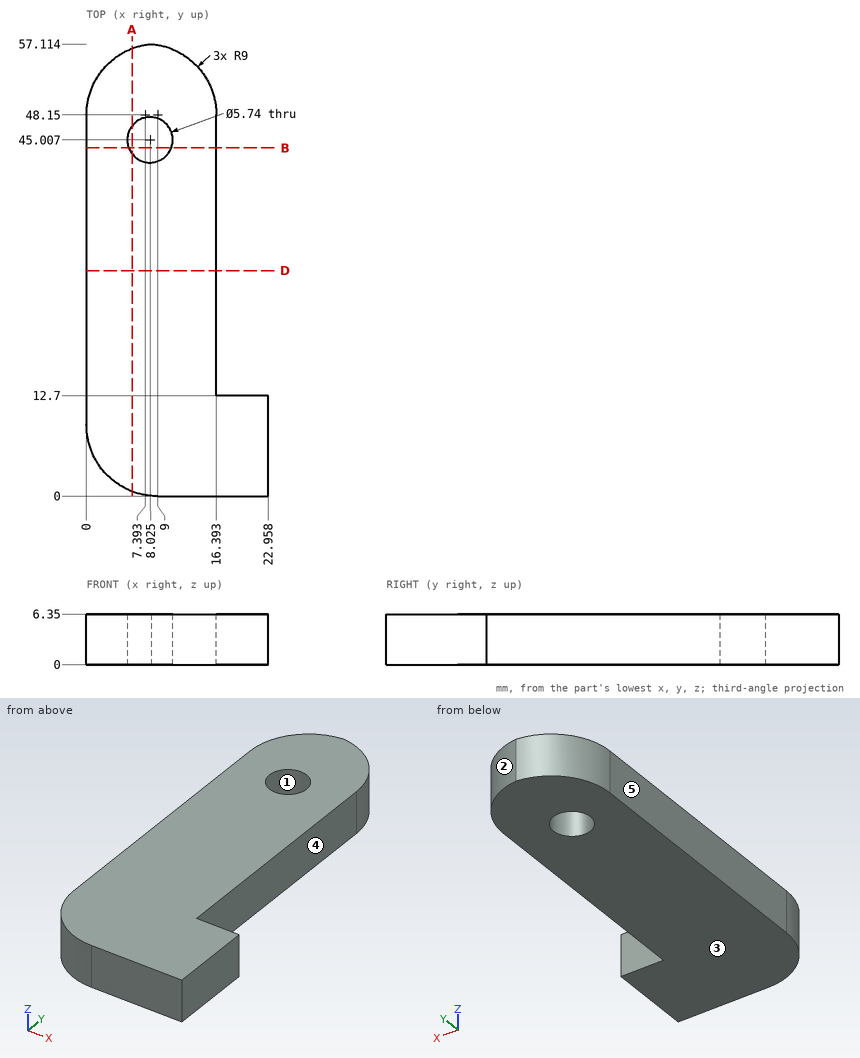
Job drawing, mm, ordinate dimensions from the low corner. One solid piece. A direction names the side the tool comes from. Coordinates: 2 decimals unless noted, no trailing zeros. Order: outer loops, then holes, each group sorted by start corner. A loop starts at its lowest first (then second) coordinate and runs counter-clockwise, first axis right, second up. Notation, with made-up numbers: (30.5, -14.5) -> (57.5, -14.5) arc R11 ccw to (57.5, 3.5) -> close; hole circle Ø5 at (43.5, 31). An arc over 180 degrees is marked (long way). Answer in a Markdown table with one row per item. Add a question column.
Q1. Mould opens along Y. For the marked faces 1, 2 and 3 say: +Y half, -Y half, draft (parallel to the pull), parting line (faces both ways), or undercut.
Q2. Band-saw the part on B-B, the plane y = 44. List the corners of the cut face in (x, z).
Q3. Wall check: line 1 along Y through (x, z) = (10.5, 5.5) (1 decimal); line 2 along Y through (x, z) = (20.5, 4); line 3 along X through (y, z) = (25.5, 4.75). Give the ranges that are in metal, low to high. Write a range as [from, to].
Q4. Band-saw the part on A-A, the plane x = 5.75. List the corners of the cut face in (y, z), then the cut area to 3 significant figures.
Q5. Drop flat-ended pins along their axis: pin 1 (1.5 mm diameter, centred on y = 24, z = 5.5, fed in from -X); pin 2 (3 mm diameter, centred on x = 19, z = 4, fed in from +Y); pin 3 (2 mm diameter, centred on x = 6.5, z = 4.5, fed in from +Y); pin 4 (1.9 mm diameter, centred on y = 36.5, z = 3, fed in from +X). Give the stop position or say it passes through.
Q6. Band-saw the part on D-D, the plane y = 28.5. List the corners of the cut face in (x, z).
Q7. Which spindle directions (+Z, -Z, +X, -X, +Y, -Y) get a long thin tool onto all of the face, cutting with end or side? Do the marked faces 4 and 5. Say none if no direction does.
Answers follow:
| question | item | result |
|---|---|---|
| 1 | face 1 | undercut |
| 1 | face 2 | +Y half |
| 1 | face 3 | draft |
| 2 | outline | (0, 0) -> (5.34, 0) -> (5.34, 6.35) -> (0, 6.35) -> close; (10.71, 0) -> (16.39, 0) -> (16.39, 6.35) -> (10.71, 6.35) -> close |
| 3 | line 1 | [0, 43.6], [46.5, 56.6] |
| 3 | line 2 | [0, 12.7] |
| 3 | line 3 | [0, 16.39] |
| 4 | outline | (0.61, 0) -> (43.26, 0) -> (43.26, 6.35) -> (0.61, 6.35) -> close; (46.76, 0) -> (56.54, 0) -> (56.54, 6.35) -> (46.76, 6.35) -> close |
| 4 | area | 333 mm^2 |
| 5 | pin 1 | x = 0 |
| 5 | pin 2 | y = 12.7 |
| 5 | pin 3 | y = 57.02 |
| 5 | pin 4 | x = 16.39 |
| 6 | outline | (0, 0) -> (16.39, 0) -> (16.39, 6.35) -> (0, 6.35) -> close |
| 7 | face 4 | +Z, -Z, +X, +Y |
| 7 | face 5 | +Z, -Z, -X, +Y, -Y |
